Check sheet for the modelled part. Datum: model origin and axes. Units: mm. A direction names the side the tool comes from. Coordinates: 2 decimals unless noted, no trailing zeros. Write each loop counter-clockwise with the first axis right and the second up, starting at its lowest first coordinate (ties: lowest second). Pieces come first, ordered by that corner, then holes. Notation, with made-up numbers: M -12.5,46.5 L -5.5,46.5 A20 cw -5.5,60.5 Z; hole C 78.25,-32.75 d9. An arc over 180 degrees is marked long. Answer as CSV lines item,"result". Start each with the question number.
1) Section check B-B (x = 9.5). Record the cut outline in (y, z), and give its area (3 significant figures).
2) Section check D-D (x = -2.5). Record the cut outline in (y, z), and give its area (3 significant figures).
3) Material ranges on L1, parallel to X at y = 0.5, z = 101; L2, parallel to Z at x = 11.5, y = 2.25; L3, parallel to X at y = -3.25, z = 121, recorded low to high. Write a range as [from, to].
4) Section check A-A (y = -1.25). Record the cut outline in (x, z).
5) Go/stop test with flat-tipped pins: pin 1 Ø3.5 at (y, z) = (0, 89.5) entering from +X; pin 2 Ø4 at (x, z) = (2.5, 103.5) entering from +Y. Record where each tip stops, or that it passes through.
6) Section check C-C (z = 188). Record the cut outline in (x, y).
7) Access from +Z, -Z, +X, -X, +Y, -Y to the whole of each face (thin tool, end or side, straight path). Record for faces 1 (the flat face through (3.5, 0, 104)), 2 (the cylindrical face through (-5, 0, 108)), 3 (the flat face through (7, 0, 220)).
from build123d import *

# Parameters (mm, degrees)
RESSALTO_EXTRUS_O1_DEPTH = 220
ESBO_O2_W                = 10
ESBO_O2_H                = 10
RESSALTO_EXTRUS_O2_DEPTH = 20


with BuildPart() as part:
    # Esboço1 → Ressalto-extrusão1 (new body)
    with BuildSketch(Plane.XY):
        with BuildLine():
            ThreePointArc((3.5, 3.570714214), (-5, 0), (3.5, -3.570714214))
            Line((3.5, -3.570714214), (3.5, 3.570714214))
        make_face()
    extrude(amount=RESSALTO_EXTRUS_O1_DEPTH)

    # Esboço2 → Ressalto-extrusão2 (add)
    with BuildSketch(Plane(origin=(0, 0, 0), x_dir=(0, 0, -1), z_dir=(1, 0, 0))):
        with Locations((-215, 0)):
            Rectangle(ESBO_O2_W, ESBO_O2_H)
    extrude(amount=RESSALTO_EXTRUS_O2_DEPTH)


solid = part.part
Results found:
1,outline,"M -5,210 L 5,210 L 5,220 L -5,220 Z"
1,area,"100 mm2"
2,outline,"M -4.33,0 L 4.33,0 L 4.33,220 L -4.33,220 Z"
2,area,"1,910 mm2"
3,L1,"x = [-4.97, 3.5]"
3,L2,"z = [210, 220]"
3,L3,"x = [-3.8, 3.5]"
4,outline,"M -4.84,0 L 3.5,0 L 3.5,210 L 20,210 L 20,220 L -4.84,220 Z"
5,pin 1,"stops at x = 3.5"
5,pin 2,"stops at y = 4.97"
6,outline,"M 3.5,-3.57 L 3.5,3.57 A5 ccw long Z"
7,face 1,"-Z, +X, +Y, -Y"
7,face 2,"-Z"
7,face 3,"+Z, +X, -X, +Y, -Y"
